```python
from build123d import *

# Parameters (mm, degrees)
SKETCH1_W           = 25
SKETCH1_H           = 25
BOSS_EXTRUDE1_DEPTH = 6
SKETCH2_R           = 8.05
CUT_EXTRUDE1_DEPTH  = 5.5
BOSS_EXTRUDE2_DEPTH = 25
SKETCH5_R           = 2.2
CUT_EXTRUDE3_DEPTH  = 7.5
SKETCH6_R           = 8.05
SKETCH6_R_2         = 5.25
BOSS_EXTRUDE3_DEPTH = 0.2
FILLET1_R           = 1
CHAMFER1_SIZE       = 0.5
CHAMFER2_SIZE       = 0.25


with BuildPart() as part:
    # Sketch1 → Boss-Extrude1 (new body)
    with BuildSketch(Plane(origin=(0, 0, 0), x_dir=(1, 0, 0), z_dir=(0, 1, 0))):
        Rectangle(SKETCH1_W, SKETCH1_H)
    extrude(amount=BOSS_EXTRUDE1_DEPTH)

    # Sketch2 → Cut-Extrude1 (cut)
    with BuildSketch(Plane(origin=(0, 6, 0), x_dir=(1, 0, 0), z_dir=(0, 1, 0))):
        with Locations((0, -3.5)):
            Circle(SKETCH2_R)
    extrude(amount=-CUT_EXTRUDE1_DEPTH, mode=Mode.SUBTRACT)

    # Sketch4 → Boss-Extrude2 (add)
    with BuildSketch(Plane.XY.offset(12.5)):
        Polygon((12.5, 4.5), (14.5, 4.5), (14.5, 3), (12.5, 1), align=None)
        Polygon((-12.5, 1), (-12.5, 4.5), (-14.5, 4.5), (-14.5, 3), align=None)
    extrude(amount=-BOSS_EXTRUDE2_DEPTH)

    # Sketch5 → Cut-Extrude3 (cut)
    with BuildSketch(Plane(origin=(0, 0, -12.5), x_dir=(-1, 0, 0), z_dir=(0, 0, -1))):
        with Locations((0, 3)):
            Circle(SKETCH5_R)
    extrude(amount=-CUT_EXTRUDE3_DEPTH, mode=Mode.SUBTRACT)

    # Sketch6 → Boss-Extrude3 (add)
    with BuildSketch(Plane(origin=(0, 0.5, 0), x_dir=(1, 0, 0), z_dir=(0, 1, 0))):
        with Locations((0, -3.5)):
            Circle(SKETCH6_R)
        with Locations((0, -3.5)):
            Circle(SKETCH6_R_2, mode=Mode.SUBTRACT)
    extrude(amount=BOSS_EXTRUDE3_DEPTH)

    # Fillet1
    fillet1_edges = [part.edges().sort_by_distance(p)[0] for p in [
        (12.5, 0.5, -12.5),
        (12.5, 0.5, 12.5),
        (13.5, 2, 12.5),
        (14.5, 3.75, 12.5),
        (14.5, 3.75, -12.5),
        (13.5, 2, -12.5),
        (-12.5, 0.5, 12.5),
        (-12.5, 0.5, -12.5),
        (-13.5, 2, 12.5),
        (-14.5, 3.75, 12.5),
        (-13.5, 2, -12.5),
        (-14.5, 3.75, -12.5),
        (12.5, 5.25, 12.5),
        (-12.5, 5.25, 12.5),
        (-12.5, 5.25, -12.5),
        (12.5, 5.25, -12.5),
    ]]
    fillet(fillet1_edges, radius=FILLET1_R)

    # Chamfer1
    chamfer1_edges = [part.edges().sort_by_distance(p)[0] for p in [
        (2.2, 3, -12.5),
    ]]
    chamfer(chamfer1_edges, length=CHAMFER1_SIZE)

    # Chamfer2
    chamfer2_edges = [part.edges().sort_by_distance(p)[0] for p in [
        (-8.05, 6, 3.5),
        (0, 0, 12.5),
        (0, 6, 12.5),
        (0, 0, -12.5),
        (0, 6, -12.5),
        (12.5, 0, 0),
        (-12.5, 0, 0),
        (12.207106781, 0, -12.207106781),
        (-12.207106781, 0, -12.207106781),
        (-12.207106781, 0, 12.207106781),
        (12.207106781, 0, 12.207106781),
        (12.5, 6, 0),
        (-12.5, 6, 0),
        (12.207106781, 6, -12.207106781),
        (-12.207106781, 6, -12.207106781),
        (-12.207106781, 6, 12.207106781),
        (12.207106781, 6, 12.207106781),
    ]]
    chamfer(chamfer2_edges, length=CHAMFER2_SIZE)


solid = part.part
```
Geometry: final body of the model. Coordinates: model frame, mm. A direction names the side the tool comes from. Coordinates: 2 decimals unless noted, no trailing zeros. Order: outer loops, then holes, each group sorted by start corner. A loop starts at its lowest first (then second) coordinate and runs counter-clockwise, first axis right, second up. Notation, with made-up numbers: M 75,40.25 L 106,40.25 A32 ccw 106,79.25 Z; hole C 83,73.25 d6. An arc over 180 degrees is marked long. Answer in a Markdown table with one row per item. Add a question column.
Q1. Reachability of faces 4 (the cylindrical face through (-12.215, 5.134, 12.199)), 5 (the cylindrical face through (-12.199, 0.711, 12.215)), 6 (the cylindrical face through (-1.745, 3.26, 11.359)) from +Z, -Z, +X, -X, +Y, -Y: full face, straight path, thin tool, end or side. Return the list, or none.
Q2. Line query: L1, parallel to Z at x = 0, y = 3; L2, parallel to X at y = 3.4, z = 3.5; L3, parallel to Y at x = 0, z = -8.25. Output: solid intervals per line, ascending.
Q3. Contact query for flat-ended pins moving along their axis: P1, Ø1.5, axis at x = 13.5, z = -3, coming from the +Y side; P2, Ø0.8, axis at y = 0.5, z = 4.5, coming from the +X side; P3, Ø8.5, axis at x = -2.5, z = 6, coming from the +Y side. Output: stop coordinate, or through.
Q4. Section query A-A on z = 3.5. Return the cut outline in (x, y).
Q5. Section query B-B on z = -8.5. Return the cut outline in (x, y), and give its area (3 significant figures).
Q6. Mould query, pull axis X, two halves, no side actions, for faces 1 (the flat face through (0, 3, -5)), 2 (the flat face through (0, 6, -6)), 3 (the flat face through (13.5, 2, 0.2)). Classes: released by +X, released by -X, zero draft, split by the parting line, or undercut.
Completed:
| question | item | result |
|---|---|---|
| 1 | face 4 | +Z, -X, +Y |
| 1 | face 5 | +Z, -X, -Y |
| 1 | face 6 | +Y |
| 2 | L1 | z = -5 to -4.55, 11.55 to 12.5 |
| 2 | L2 | x = -14.5 to -8.05, 8.05 to 14.5 |
| 2 | L3 | y = 0 to 0.8, 5.2 to 6 |
| 3 | P1 | stops at y = 4.5 |
| 3 | P2 | stops at x = 12.5 |
| 3 | P3 | stops at y = 0.7 |
| 4 | outline | M -14.5,3 L -12.5,1 L -12.5,0.25 L -12.25,0 L 12.25,0 L 12.5,0.25 L 12.5,1 L 14.5,3 L 14.5,4.5 L 12.5,4.5 L 12.5,5.75 L 12.25,6 L 8.3,6 L 8.05,5.75 L 8.05,0.7 L 5.25,0.7 L 5.25,0.5 L -5.25,0.5 L -5.25,0.7 L -8.05,0.7 L -8.05,5.75 L -8.3,6 L -12.25,6 L -12.5,5.75 L -12.5,4.5 L -14.5,4.5 Z |
| 5 | outline | M -14.5,3 L -12.5,1 L -12.5,0.25 L -12.25,0 L 12.25,0 L 12.5,0.25 L 12.5,1 L 14.5,3 L 14.5,4.5 L 12.5,4.5 L 12.5,5.75 L 12.25,6 L -12.25,6 L -12.5,5.75 L -12.5,4.5 L -14.5,4.5 Z; hole C 0,3 d4.4 |
| 5 | area | 145 mm2 |
| 6 | face 1 | undercut |
| 6 | face 2 | zero draft |
| 6 | face 3 | released by +X |
